For this review, take the finished solid that the model builds, in its own axes (mm). A direction names the side the tool comes from. Coordinates: 2 decimals unless noted, no trailing zeros. Loops run counter-clockwise (first coordinate to the right, second up) from the corner with the lowest first, then second, coordinate; pieces in that order, holes last. Notation, with made-up numbers: M -37.5,-8.5 L -10.5,-8.5 A18 cw -10.5,10.5 Z; hole C 46,-34 d4. An arc over 180 degrees is marked long. Answer as a JSON object with one key per item and string values. Group by question number.
Item 1: Tool access review of faces 1 (the face through (17, -20.869, -6)), 2 (the face through (17, -28.869, -6)), 3 (the face through (15, -31.869, -8)): name each direction out of +Z, -Z, +X, -X, +Y, -Y from which nothing blocks a thin tool from reaching the whole face with its end or side.
Item 2: Add section B-B (z = -13). State the section outline as (x, y) points, then the cut area to 3 significant figures.
Item 3: Add section C-C (x = 6.5). State the section outline as (y, z) points.
Item 4: Insertion check: pin 1 (2 mm diameter, centred on y = -25, z = -9, fed in from +X); pin 2 (4 mm diameter, centred on x = 14.5, z = -4, fed in from +Y); pin 3 (3 mm diameter, centred on x = 12.5, z = -13.5, fed in from +Y). Each pin has a flat end and moves straight along its axis. Give the tip position at first contact, or say it passes through.
Item 5: Add section D-D (x = 18). State the section outline as (y, z) points.
Item 6: Wall thickness on L1, parallel to Y at x = 16.5, z = -5; L2, parallel to X at y = 11, z = -11; L3, parallel to X at y = -23.5, z = -9.75: over which ranges is each line inside the solid? List them lowest first. Write a range as from..to.
Item 7: Add section A-A (z = -8). State the section outline as (x, y) points.
Item 8: Mouldability with a two-part tool opening along X and no side actions: class faces 4 (the face through (-16.058, -7, -8)), 5 (the face through (-1, -6, 0)), 6 (the face through (11.942, -25, -8)), 7 (the face through (18.58, -22.35, -8.21)) as +X half, -X half, draft (parallel to the pull), parting line (faces both ways), or undercut.
from build123d import *

# Parameters (mm, degrees)
SKETCH1_R           = 4.15
BOSS_EXTRUDE1_DEPTH = 16
SKETCH2_R           = 4.15
CUT_EXTRUDE1_DEPTH  = 63.237043653
SKETCH3_R           = 1.65
CUT_EXTRUDE2_DEPTH  = 51.435102881


with BuildPart() as part:
    # Sketch1 → Boss-Extrude1 (new body)
    with BuildSketch(Plane.XY):
        with BuildLine():
            Line((11.941959863, -20.868835105), (21.941959863, -20.868835105))
            Line((21.941959863, -20.868835105), (21.941959863, -23.868835105))
            Line((21.941959863, -23.868835105), (11.941959863, -23.868835105))
            Line((11.941959863, -23.868835105), (11.941959863, -26.368835105))
            ThreePointArc((11.941959863, -26.368835105), (11.841160348, -27.63478601), (11.541301939, -28.868835105))
            Line((11.541301939, -28.868835105), (21.941959863, -28.868835105))
            Line((21.941959863, -28.868835105), (21.941959863, -31.868835105))
            Line((21.941959863, -31.868835105), (9.751434882, -31.868835105))
            ThreePointArc((9.751434882, -31.868835105), (7.104237523, -33.717304334), (3.941959863, -34.368835105))
            Line((3.941959863, -34.368835105), (-16.058040137, -34.368835105))
            Line((-16.058040137, -34.368835105), (-16.058040137, 21.631164895))
            Line((-16.058040137, 21.631164895), (3.941959863, 21.631164895))
            ThreePointArc((3.941959863, 21.631164895), (9.598814112, 19.288019144), (11.941959863, 13.631164895))
            Line((11.941959863, 13.631164895), (11.941959863, -20.868835105))
        make_face()
        with Locations((3.941959863, 13.631164895)):
            Circle(SKETCH1_R, mode=Mode.SUBTRACT)
        with Locations((3.941959863, -26.368835105)):
            Circle(SKETCH1_R, mode=Mode.SUBTRACT)
    extrude(amount=-BOSS_EXTRUDE1_DEPTH)

    # Sketch2 → Cut-Extrude1 (cut, through all)
    with BuildSketch(Plane(origin=(0, 21.631164895, 0), x_dir=(1, 0, 0), z_dir=(0, 1, 0))):
        with Locations(Location((-8.058040137, 8, 0), (0, 0, 270))):
            Circle(SKETCH2_R)
    extrude(amount=-CUT_EXTRUDE1_DEPTH, mode=Mode.SUBTRACT)

    # Sketch3 → Cut-Extrude2 (cut, through all)
    with BuildSketch(Plane(origin=(0, -20.868835105, 0), x_dir=(1, 0, 0), z_dir=(0, 1, 0))):
        with Locations(Location((16.941959863, 8, 0), (0, 0, 270))):
            Circle(SKETCH3_R)
    extrude(amount=-CUT_EXTRUDE2_DEPTH, mode=Mode.SUBTRACT)


solid = part.part
From the geometry:
{
 "1": {"face 1": "+Z, -Z, +X, +Y", "face 2": "+Z, -Z, +X", "face 3": "+Z, -Z, +X, -Y"},
 "2": {"outline": "M -16.06,-34.37 L 3.94,-34.37 A8 ccw 9.75,-31.87 L 21.94,-31.87 L 21.94,-28.87 L 11.54,-28.87 A8 ccw 11.94,-26.37 L 11.94,-23.87 L 21.94,-23.87 L 21.94,-20.87 L 11.94,-20.87 L 11.94,13.63 A8 ccw 3.94,21.63 L -16.06,21.63 Z; hole C 3.94,-26.37 d8.3; hole C 3.94,13.63 d8.3", "area": "1,500 mm²"},
 "3": {"outline": "M -33.95,-16 L -29.64,-16 L -29.64,0 L -33.95,0 Z; M -23.1,-16 L 10.36,-16 L 10.36,0 L -23.1,0 Z; M 16.9,-16 L 21.21,-16 L 21.21,0 L 16.9,0 Z"},
 "4": {"pin 1": "stops at x = 11.94", "pin 2": "stops at y = -20.87", "pin 3": "stops at y = 17.4"},
 "5": {"outline": "M -31.87,-16 L -28.87,-16 L -28.87,-9.27 L -31.87,-9.27 Z; M -31.87,-6.73 L -28.87,-6.73 L -28.87,0 L -31.87,0 Z; M -23.87,-16 L -20.87,-16 L -20.87,-9.27 L -23.87,-9.27 Z; M -23.87,-6.73 L -20.87,-6.73 L -20.87,0 L -23.87,0 Z"},
 "6": {"L1": "y = -31.87..-28.87, -23.87..-20.87", "L2": "x = -16.06..-10.93, -5.19..0.73, 7.15..11.94", "L3": "x = -16.06..-11.82, -4.3..0.94, 6.94..21.94"},
 "7": {"outline": "M -16.06,-34.37 L -12.21,-34.37 L -12.21,21.63 L -16.06,21.63 Z; M -3.91,-34.37 L 3.94,-34.37 A8 ccw 9.75,-31.87 L 15.29,-31.87 L 15.29,-28.87 L 11.54,-28.87 A8 ccw 11.94,-26.37 L 11.94,-23.87 L 15.29,-23.87 L 15.29,-20.87 L 11.94,-20.87 L 11.94,13.63 A8 ccw 3.94,21.63 L -3.91,21.63 Z; M 18.59,-31.87 L 21.94,-31.87 L 21.94,-28.87 L 18.59,-28.87 Z; M 18.59,-23.87 L 21.94,-23.87 L 21.94,-20.87 L 18.59,-20.87 Z; hole C 3.94,-26.37 d8.3; hole C 3.94,13.63 d8.3"},
 "8": {"face 4": "-X half", "face 5": "draft", "face 6": "+X half", "face 7": "undercut"}
}
